```python
from build123d import *

# Parameters (mm, degrees)
SKETCH1_W           = 67.5
SKETCH1_H           = 53
SKETCH1_R           = 1.75
SKETCH1_W_2         = 7.5
BOSS_EXTRUDE1_DEPTH = 1.5
CUT_EXTRUDE1_DEPTH  = 2
FILLET1_R           = 1
FILLET2_R           = 2
SKETCH3_W           = 7.5
SKETCH3_H           = 9
CUT_EXTRUDE2_DEPTH  = 2
BOSS_EXTRUDE2_DEPTH = 11
SKETCH5_W           = 7.5
SKETCH5_H           = 12
CUT_EXTRUDE3_DEPTH  = 1.5
SKETCH6_W           = 3
SKETCH6_H           = 5.5
CUT_EXTRUDE4_DEPTH  = 12
BOSS_EXTRUDE3_DEPTH = 11
SKETCH8_W           = 2
SKETCH8_H           = 9
CUT_EXTRUDE5_DEPTH  = 1.5
SKETCH9_R           = 3
SKETCH9_R_2         = 0.75
CUT_EXTRUDE6_DEPTH  = 9
SKETCH10_R          = 0.75
CUT_EXTRUDE7_DEPTH  = 2
FILLET3_R           = 0.75
CUT_EXTRUDE8_DEPTH  = 10


with BuildPart() as part:
    # Sketch1 → Boss-Extrude1 (new body)
    with BuildSketch(Plane.XY):
        with Locations((-3.75, 0)):
            Rectangle(SKETCH1_W, SKETCH1_H)
        with Locations((-35.25, -8.5)):
            Circle(SKETCH1_R, mode=Mode.SUBTRACT)
        with Locations((16, -24.25)):
            Circle(SKETCH1_R, mode=Mode.SUBTRACT)
        with Locations((-35.25, 19)):
            Circle(SKETCH1_R, mode=Mode.SUBTRACT)
        with Locations((16, 24.25)):
            Circle(SKETCH1_R, mode=Mode.SUBTRACT)
        with Locations((33.75, 0)):
            Rectangle(SKETCH1_W_2, SKETCH1_H)
    extrude(amount=BOSS_EXTRUDE1_DEPTH)

    # Sketch2 → Cut-Extrude1 (cut)
    with BuildSketch(Plane.XY.offset(1.5)):
        Polygon((-37.5, 26.5), (-37.5, 21.544210715), (-35.5, 23.131873366), (-35.5, 26.5), align=None)
        Polygon((-37.5, -11.044210715), (-37.5, -26.5), (-35.5, -26.5), (-35.5, -16), (-35.5, -12.631873366), align=None)
    extrude(amount=-CUT_EXTRUDE1_DEPTH, mode=Mode.SUBTRACT)

    # Fillet1
    fillet1_edges = [part.edges().sort_by_distance(p)[0] for p in [
        (-35.5, 23.131873366, 0.75),
        (-37.5, 21.544210715, 0.75),
        (-35.5, -12.631873366, 0.75),
        (-37.5, -11.044210715, 0.75),
    ]]
    fillet(fillet1_edges, radius=FILLET1_R)

    # Fillet2
    fillet2_edges = [part.edges().sort_by_distance(p)[0] for p in [
        (-35.5, 26.5, 0.75),
        (-35.5, -26.5, 0.75),
    ]]
    fillet(fillet2_edges, radius=FILLET2_R)

    # Sketch3 → Cut-Extrude2 (cut)
    with BuildSketch(Plane.XY.offset(1.5)):
        Polygon((30, -5.5), (37.5, -5.5), (37.5, 26.5), (30, 26.5), (30, 23.5), (32, 23.5), (32, 14.5), (30, 14.5), align=None)
        with Locations((33.75, -22)):
            Rectangle(SKETCH3_W, SKETCH3_H)
    extrude(amount=-CUT_EXTRUDE2_DEPTH, mode=Mode.SUBTRACT)

    # Sketch4 → Boss-Extrude2 (add)
    with BuildSketch(Plane.XY.offset(1.5)):
        Polygon((37.5, -17.5), (30, -17.5), (21.5, -17.5), (21.5, -5.5), (30, -5.5), (37.5, -5.5), align=None)
    extrude(amount=BOSS_EXTRUDE2_DEPTH)

    # Sketch5 → Cut-Extrude3 (cut)
    with BuildSketch(Plane(origin=(0, 0, 0), x_dir=(-1, 0, 0), z_dir=(0, 0, -1))):
        with Locations((-33.75, -11.5)):
            Rectangle(SKETCH5_W, SKETCH5_H)
    extrude(amount=-CUT_EXTRUDE3_DEPTH, mode=Mode.SUBTRACT)

    # Sketch6 → Cut-Extrude4 (cut)
    with BuildSketch(Plane(origin=(37.5, 0, 0), x_dir=(0, 0, -1), z_dir=(1, 0, 0))):
        Polygon((-3, -16.5), (-3, -6.5), (-9.334936491, -6.5), (-11.5, -9.25), (-11.5, -13.75), (-9.334936491, -16.5), align=None)
        with Locations((-7, -11.5)):
            Rectangle(SKETCH6_W, SKETCH6_H, mode=Mode.SUBTRACT)
    extrude(amount=-CUT_EXTRUDE4_DEPTH, mode=Mode.SUBTRACT)

    # Sketch7 → Boss-Extrude3 (add)
    with BuildSketch(Plane.XY.offset(1.5)):
        Polygon((32, 14.5), (30, 14.5), (19, 14.5), (19, 23.5), (30, 23.5), (32, 23.5), align=None)
    extrude(amount=BOSS_EXTRUDE3_DEPTH)

    # Sketch8 → Cut-Extrude5 (cut)
    with BuildSketch(Plane(origin=(0, 0, 0), x_dir=(-1, 0, 0), z_dir=(0, 0, -1))):
        with Locations((-31, 19)):
            Rectangle(SKETCH8_W, SKETCH8_H)
    extrude(amount=-CUT_EXTRUDE5_DEPTH, mode=Mode.SUBTRACT)

    # Sketch9 → Cut-Extrude6 (cut)
    with BuildSketch(Plane(origin=(32, 0, 0), x_dir=(0, 0, -1), z_dir=(1, 0, 0))):
        with Locations((-8, 19)):
            Circle(SKETCH9_R)
        with Locations((-8, 19)):
            Circle(SKETCH9_R_2, mode=Mode.SUBTRACT)
    extrude(amount=-CUT_EXTRUDE6_DEPTH, mode=Mode.SUBTRACT)

    # Sketch10 → Cut-Extrude7 (cut)
    with BuildSketch(Plane(origin=(32, 0, 0), x_dir=(0, 0, -1), z_dir=(1, 0, 0))):
        with Locations((-8, 19)):
            Circle(SKETCH10_R)
    extrude(amount=-CUT_EXTRUDE7_DEPTH, mode=Mode.SUBTRACT)

    # Fillet3
    fillet3_edges = [part.edges().sort_by_distance(p)[0] for p in [
        (30, 19, 8.75),
    ]]
    fillet(fillet3_edges, radius=FILLET3_R)

    # Sketch11 → Cut-Extrude8 (cut)
    with BuildSketch(Plane.ZY.offset(-19)):
        with BuildLine():
            Line((8, 14.5), (12.5, 14.5))
            Line((12.5, 14.5), (12.5, 23.5))
            Line((12.5, 23.5), (8, 23.5))
            Line((8, 23.5), (8, 23))
            ThreePointArc((8, 23), (12, 19), (8, 15))
            Line((8, 15), (8, 14.5))
        make_face()
    extrude(amount=-CUT_EXTRUDE8_DEPTH, mode=Mode.SUBTRACT)


solid = part.part
```
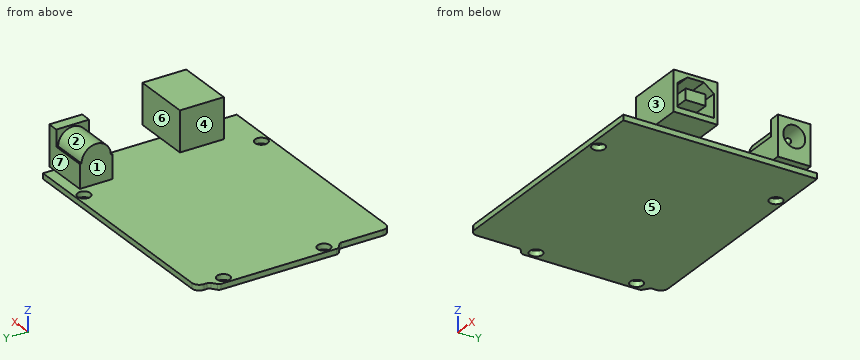
Design review of the part built by this model. Coordinates are the model's own, in mm. Face numbers are marked on the shaded views. A direction names the side the tool comes from. Give positions to 0.01 mm unless a question says otherwise; leave off trailing zeros. Order: outer loops, then holes, each group sorted by start corner. A loop starts at its lowest first (then second) coordinate and runs counter-clockwise, first axis right, second up. Notation, with made-up numbers: (48.5, 42.5) -> (93.5, 42.5) arc R16 ccw to (93.5, 54.5) -> close; hole circle Ø8 at (-8, 7.25). An arc over 180 degrees is marked (long way). Write each question's results on one line, items separated by ' | '. Start each with the question number.
Q1. Machinability: for the marked faces 1, 2, 3 and 4, which of the approach directions +Z, -Z, +X, -X, +Y, -Y give a long, thin tool a straight path to every point of the face, cutting with its end or side? Answer none if there is none.
Q2. Add section A-A on z = 3.75. Give the boundary of the cut face in (x, y).
Q3. Mouldability with a two-part tool opening along Y and no side actions: class the marked faces 5, 6 and 7 as +Y half, -Y half, draft (parallel to the pull), parting line (faces both ways), or undercut.
Q4. For pin 1 (6 mm diameter, centred on x = 9, z = 6.5, fed in from +Y); pin 2 (1.5 mm diameter, centred on x = 33, z = 6.5, fed in from -Y); pin 3 (7 mm diameter, centred on y = 19, z = 8, fed in from +X); pin 4 (1.9 mm diameter, centred on x = 30.5, z = 7.5, fed in from +Y), all flat-tipped, find the tip position at first contact; note any pin that passes through.
Q5. Add section C-C on y = -1. Give the boundary of the cut face in (x, z).
Q6. Wall thickness on L1, parallel to Y at x = 29.5, z = 8; L2, parallel to Z at x = -9, y = -14.5; L3, parallel to X at y = 11, z = 1.25: over which ranges is each line inside the solid? List them lowest first. Write a range as from..to.
Q7. Add section D-D on x = -3. Give the boundary of the cut face in (y, z), and give its area (3 significant figures).
Q8. Add section B-B on x = 16. Give the boundary of the cut face in (y, z), and give its area (3 significant figures).
Found:
1) face 1: +Z, -X, +Y, -Y | face 2: +Z, -X | face 3: +Z, +X, -X, -Y | face 4: +Z, -X, -Y
2) outline: (19, 14.5) -> (32, 14.5) -> (32, 23.5) -> (19, 23.5) -> close; (21.5, -17.5) -> (37.5, -17.5) -> (37.5, -16.5) -> (25.5, -16.5) -> (25.5, -6.5) -> (37.5, -6.5) -> (37.5, -5.5) -> (21.5, -5.5) -> close
3) face 5: draft | face 6: undercut | face 7: +Y half
4) pin 1: passes through | pin 2: stops at y = -17.5 | pin 3: stops at x = 32 | pin 4: stops at y = 23.5
5) outline: (-37.5, 0) -> (30, 0) -> (30, 1.5) -> (-37.5, 1.5) -> close
6) L1: y = -17.5..-16.5, -14.25..-8.75, -6.5..-5.5, 14.5..16, 18.29..19.71, 22..23.5 | L2: z = 0..1.5 | L3: x = -37.5..30
7) outline: (-26.5, 0) -> (26.5, 0) -> (26.5, 1.5) -> (-26.5, 1.5) -> close | area: 79.5 mm2
8) outline: (-26.5, 0) -> (-26, 0) -> (-26, 1.5) -> (-26.5, 1.5) -> close; (-22.5, 0) -> (22.5, 0) -> (22.5, 1.5) -> (-22.5, 1.5) -> close; (26, 0) -> (26.5, 0) -> (26.5, 1.5) -> (26, 1.5) -> close | area: 69.0 mm2
